The model under review builds one solid part; all positions refer to its coordinate system, in mm. Round coordinates to 2 decimals unless told otherwise and drop trailing zeros. Order: outer loops, then holes, each group sorted by start corner. A loop starts at its lowest first (then second) coordinate and runs counter-clockwise, first axis right, second up. Notation, with made-up numbers: M 29.25,31.25 L 36.25,31.25 A15 cw 36.25,45.25 Z; hole C 73.5,-5 d8. An arc over 180 degrees is marked long. Use a Markdown table: item, result. Add a question column.
1. Consider section A-A on z = 33.25. State the section outline as (x, y) points, then the cut area to 3 significant figures.
2. Consider section B-B on x = -49.75. State the section outline as (y, z) points, then the cut area to 3 significant figures.
3. To check wall thickness, follow probe 1 along X at (y, z) = (-92.75, 31.25); probe 2 along Z at (x, y) = (-51, -94.75); probe 3 along Z at (x, y) = (-47.25, -93.25). State the ranges of each line that lie inside material, in increasing order.
4. Insertion check: P1, Ø6, axis at x = -59, z = 43.5, coming from the -Y side; P2, Ø4, axis at x = -46, z = 47, coming from the -Y side; P3, Ø6, axis at x = -62, z = 29, coming from the -Y side; P4, Ø3, axis at y = -94, z = 47.5, coming from the +X side. Each pin has a flat end and moves straight along its axis. Give the tip position at first contact, or say it passes through.
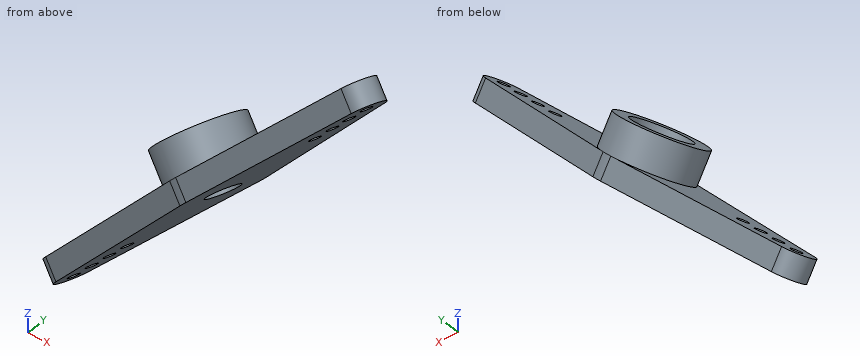
from build123d import *
from build123d.topology import SkipClean

# Parameters (mm, degrees)
SKETCH1_R           = 1.134023506
SKETCH1_R_2         = 0.399750463
BOSS_EXTRUDE1_DEPTH = 1.4986
SKETCH2_R           = 2.9591
BOSS_EXTRUDE2_DEPTH = 2.159
SKETCH3_R           = 1.9812
CUT_EXTRUDE1_DEPTH  = 2.54


with BuildPart() as part:
    # Sketch1 → Boss-Extrude1 (new body)
    with BuildSketch(Plane(origin=(-26.118953855, 9.878989701, 23.95417966), x_dir=(0.6811926509137779, 0.027031276316117844, 0.7316050043854141), z_dir=(-0.7099227615957759, 0.26851456951758673, 0.6510834036627045))):
        with BuildLine():
            Line((-10.17960006, -104.330094763), (4.464711493, -106.277674051))
            ThreePointArc((4.464711493, -106.277674051), (5.521063626, -107.502012677), (4.428867403, -108.694485866))
            Line((4.428867403, -108.694485866), (-10.26676012, -110.206920218))
            ThreePointArc((-10.26676012, -110.206920218), (-10.569702558, -110.222468165), (-10.872644997, -110.206920218))
            Line((-10.872644997, -110.206920218), (-25.56827252, -108.694485866))
            ThreePointArc((-25.56827252, -108.694485866), (-26.660468742, -107.502012677), (-25.60411661, -106.277674051))
            Line((-25.60411661, -106.277674051), (-10.959805057, -104.330094763))
            ThreePointArc((-10.959805057, -104.330094763), (-10.569702558, -104.304268165), (-10.17960006, -104.330094763))
        make_face()
        with Locations(Location((-10.569702558, -107.263368165, 0), (0, 0, 358.39196451))):
            Circle(SKETCH1_R, mode=Mode.SUBTRACT)
        with Locations(Location((4.304284008, -107.48396644, 0), (0, 0, 358.39196451))):
            Circle(SKETCH1_R_2, mode=Mode.SUBTRACT)
        with Locations(Location((2.526284008, -107.457596661, 0), (0, 0, 358.39196451))):
            Circle(SKETCH1_R_2, mode=Mode.SUBTRACT)
        with Locations(Location((0.748284008, -107.431226882, 0), (0, 0, 358.39196451))):
            Circle(SKETCH1_R_2, mode=Mode.SUBTRACT)
        with Locations(Location((-1.029715992, -107.404857104, 0), (0, 0, 358.39196451))):
            Circle(SKETCH1_R_2, mode=Mode.SUBTRACT)
        with Locations(Location((-20.109689125, -107.404857104, 0), (0, 0, 178.39196451))):
            Circle(SKETCH1_R_2, mode=Mode.SUBTRACT)
        with Locations(Location((-21.887689125, -107.431226882, 0), (0, 0, 178.39196451))):
            Circle(SKETCH1_R_2, mode=Mode.SUBTRACT)
        with Locations(Location((-23.665689125, -107.457596661, 0), (0, 0, 178.39196451))):
            Circle(SKETCH1_R_2, mode=Mode.SUBTRACT)
        with Locations(Location((-25.443689125, -107.48396644, 0), (0, 0, 178.39196451))):
            Circle(SKETCH1_R_2, mode=Mode.SUBTRACT)
    extrude(amount=BOSS_EXTRUDE1_DEPTH)

    # Sketch2 → Boss-Extrude2 (add)
    with SkipClean():  # the faces are left unmerged after this step: merging them gives an invalid solid
        with BuildSketch(Plane(origin=(-27.182844105, 10.281385635, 24.929893249), x_dir=(0.681192650913778, 0.027031276316117795, 0.731605004385414), z_dir=(-0.7099227615957758, 0.2685145695175868, 0.6510834036627047))):
            with Locations(Location((-10.569702558, -107.263368165, 0), (0, 0, 97.575438716))):
                Circle(SKETCH2_R)
        extrude(amount=BOSS_EXTRUDE2_DEPTH)

    # Sketch3 → Cut-Extrude1 (cut)
    with SkipClean():  # the faces are left unmerged after this step: merging them gives an invalid solid
        with BuildSketch(Plane(origin=(-28.715567348, 10.861108591, 26.335582317), x_dir=(0.6811926509137781, 0.02703127631611777, 0.731605004385414), z_dir=(-0.7099227615957758, 0.26851456951758684, 0.6510834036627048))):
            with Locations(Location((-10.569702558, -107.263368165, 0), (0, 0, 358.39196451))):
                Circle(SKETCH3_R)
        extrude(amount=-CUT_EXTRUDE1_DEPTH, mode=Mode.SUBTRACT)


solid = part.part
Answer block:
| question | item | result |
|---|---|---|
| 1 | outline | M -59.58,-95.56 L -57.66,-96.05 L -56.02,-91.71 L -58.06,-91.52 Z |
| 1 | area | 8.85 mm^2 |
| 2 | outline | M -95.96,41.84 L -91.16,39.86 L -90.92,42.06 L -95.37,43.89 Z |
| 2 | area | 10.7 mm^2 |
| 3 | probe 1 | -60.36 to -58.25 |
| 3 | probe 2 | 39.97 to 42.28 |
| 3 | probe 3 | 43.45 to 45.49 |
| 4 | P1 | through |
| 4 | P2 | y = -95.39 |
| 4 | P3 | y = -95.83 |
| 4 | P4 | x = -42.37 |
